```python
from build123d import *

# Parameters (mm, degrees)
CYLINDER485_R     = 3.5
CYLINDER485_DEPTH = 4
CYLINDER484_R     = 54.5
CYLINDER484_DEPTH = 28
CYLINDER473_R     = 1.5
CYLINDER473_DEPTH = 100
CYLINDER471_R     = 1.5
CYLINDER471_DEPTH = 100
CYLINDER464_R     = 1.5
CYLINDER464_DEPTH = 100
CYLINDER466_R     = 1.5
CYLINDER466_DEPTH = 100
CYLINDER460_R     = 1.5
CYLINDER460_DEPTH = 100
CYLINDER463_R     = 1.5
CYLINDER463_DEPTH = 100
CYLINDER468_R     = 1.5
CYLINDER468_DEPTH = 100
CYLINDER470_R     = 1.5
CYLINDER470_DEPTH = 100
BOX213_W          = 10
BOX213_H          = 108
BOX213_DEPTH      = 45


with BuildPart() as obj1:
    # Cylinder485 → Cylinder485 (new body)
    with BuildSketch(Plane(origin=(50, 0, 5), x_dir=(1, 0, 0), z_dir=(0, 0, 1))):
        Circle(CYLINDER485_R)
    extrude(amount=CYLINDER485_DEPTH)


with BuildPart() as obj2:
    # Cylinder484 → Cylinder484 (new body)
    with BuildSketch(Plane.XY.offset(9)):
        Circle(CYLINDER484_R)
    extrude(amount=CYLINDER484_DEPTH)


with BuildPart() as obj3:
    # Cylinder473 → Cylinder473 (new body)
    with BuildSketch(Plane(origin=(24, -51, 25), x_dir=(0, 0, -1), z_dir=(1, 0, 0))):
        Circle(CYLINDER473_R)
    extrude(amount=CYLINDER473_DEPTH)


with BuildPart() as obj4:
    # Cylinder471 → Cylinder471 (new body)
    with BuildSketch(Plane(origin=(24, 36, 34), x_dir=(0, 0, -1), z_dir=(1, 0, 0))):
        Circle(CYLINDER471_R)
    extrude(amount=CYLINDER471_DEPTH)


with BuildPart() as obj5:
    # Cylinder464 → Cylinder464 (new body)
    with BuildSketch(Plane(origin=(24, -36, 34), x_dir=(0, 0, -1), z_dir=(1, 0, 0))):
        Circle(CYLINDER464_R)
    extrude(amount=CYLINDER464_DEPTH)


with BuildPart() as obj6:
    # Cylinder466 → Cylinder466 (new body)
    with BuildSketch(Plane(origin=(24, -23, -5), x_dir=(0, 0, -1), z_dir=(1, 0, 0))):
        Circle(CYLINDER466_R)
    extrude(amount=CYLINDER466_DEPTH)


with BuildPart() as obj7:
    # Cylinder460 → Cylinder460 (new body)
    with BuildSketch(Plane(origin=(24, 51, 7), x_dir=(0, 0, -1), z_dir=(1, 0, 0))):
        Circle(CYLINDER460_R)
    extrude(amount=CYLINDER460_DEPTH)


with BuildPart() as obj8:
    # Cylinder463 → Cylinder463 (new body)
    with BuildSketch(Plane(origin=(24, 23, -5), x_dir=(0, 0, -1), z_dir=(1, 0, 0))):
        Circle(CYLINDER463_R)
    extrude(amount=CYLINDER463_DEPTH)


with BuildPart() as obj9:
    # Cylinder468 → Cylinder468 (new body)
    with BuildSketch(Plane(origin=(24, -51, 7), x_dir=(0, 0, -1), z_dir=(1, 0, 0))):
        Circle(CYLINDER468_R)
    extrude(amount=CYLINDER468_DEPTH)


with BuildPart() as compound594:
    # Cylinder470 → Cylinder470 (new body)
    with BuildSketch(Plane(origin=(24, 51, 25), x_dir=(0, 0, -1), z_dir=(1, 0, 0))):
        Circle(CYLINDER470_R)
    extrude(amount=CYLINDER470_DEPTH)

    # Compound594: union obj3, obj4, obj5, obj6, obj7, obj8, obj9
    add(obj3.part)
    add(obj4.part)
    add(obj5.part)
    add(obj6.part)
    add(obj7.part)
    add(obj8.part)
    add(obj9.part)


with BuildPart() as cut371:
    # Box213 → Box213 (new body)
    with BuildSketch(Plane(origin=(46, -54, -8), x_dir=(1, 0, 0), z_dir=(0, 0, 1))):
        with Locations((5, 54)):
            Rectangle(BOX213_W, BOX213_H)
    extrude(amount=BOX213_DEPTH)

    # Cut374: cut Compound594
    add(compound594.part, mode=Mode.SUBTRACT)

    # Cut375: cut obj2
    add(obj2.part, mode=Mode.SUBTRACT)

    # Cut371: cut obj1
    add(obj1.part, mode=Mode.SUBTRACT)


solid = cut371.part
```
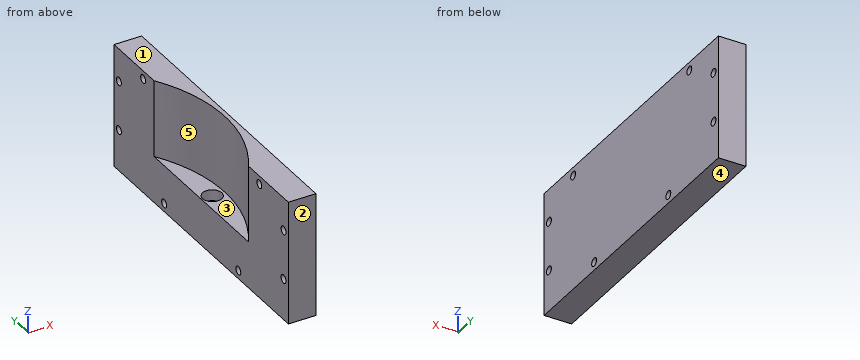
Input: part model. Units: mm. Frame: model coordinates. Face numbers are marked on the shaded views. A direction names the side the tool comes from. Give positions to 0.01 mm unless a question says otherwise; leave off trailing zeros. Order: outer loops, then holes, each group sorted by start corner. A loop starts at its lowest first (then second) coordinate and runs counter-clockwise, first axis right, second up. Notation, with made-up numbers: (45, -17.5) - (49, -17.5) arc R14 ccw to (49, -1.5) - close; hole circle Ø8 at (-30, 24). An arc over 180 degrees is marked (long way). One line per item, written item: value.
1. Cut plane D-D, the plane x = 50.5. Give the number of separate pieces and of enclosed holes in the cut face, and give its area (3 significant figures).
Determined:
separate pieces: 1
enclosed holes: 8
area: 3,630 mm2
2. Reachability of the marked faces 4 and 5 from +Z, -Z, +X, -X, +Y, -Y: full face, straight path, thin tool, end or side. Return the list, or none.
Determined:
face 4: -Z, +X, -X, +Y, -Y
face 5: +Z, -X
3. Draft query along Y for the marked faces 1, 2 and 3. Return one class per face: released by +Y, released by -Y, zero draft, split by the parting line, or undercut.
Determined:
face 1: zero draft
face 2: released by -Y
face 3: undercut
4. Cut plane B-B, the plane y = -51. Output: boundary loops of the cut face in (x, z), and give its area (3 significant figures).
Determined:
outline: (46, -8) - (56, -8) - (56, 5.5) - (46, 5.5) - close; (46, 8.5) - (56, 8.5) - (56, 23.5) - (46, 23.5) - close; (46, 26.5) - (56, 26.5) - (56, 37) - (46, 37) - close
area: 390 mm2
5. Cut plane C-C, the plane y = 36. Output: boundary loops of the cut face in (x, z), and give its area (3 significant figures).
Determined:
outline: (46, -8) - (56, -8) - (56, 32.5) - (46, 32.5) - close; (46, 35.5) - (56, 35.5) - (56, 37) - (46, 37) - close
area: 420 mm2
6. Cut plane A-A, the plane z = -5. Output: boundary loops of the cut face in (x, y).
Determined:
outline: (46, -54) - (56, -54) - (56, -24.5) - (46, -24.5) - close; (46, -21.5) - (56, -21.5) - (56, 21.5) - (46, 21.5) - close; (46, 24.5) - (56, 24.5) - (56, 54) - (46, 54) - close
7. Line query: probe 1 along Z at (x, y) = (53.25, 23); probe 2 along Y at (x, z) = (53.5, -5); probe 3 along Y at (x, z) = (48, 25). Output: solid intervals per line, ascending.
Determined:
probe 1: -8 to -6.5, -3.5 to 37
probe 2: -54 to -24.5, -21.5 to 21.5, 24.5 to 54
probe 3: -54 to -52.5, -49.5 to -25.81, 25.81 to 49.5, 52.5 to 54
8. Pin query (flat end, axial travel): pin 1 Ø2.5 at (y, z) = (-51, 7) entering from +X; pin 2 Ø2 at (x, y) = (49.5, -1) entering from +Z; pin 3 Ø2 at (x, y) = (50.5, 11) entering from +Z. Return the tip coordinate at first contact, or that it passes through.
Determined:
pin 1: through
pin 2: z = 5
pin 3: z = 9
